from build123d import *

# Parameters (mm, degrees)
BOSS_EXTRU_1_DEPTH      = 20
ESQUISSE2_W             = 4.75
ESQUISSE2_H             = 4.5
ENL_V_MAT_EXTRU_1_DEPTH = 21
ESQUISSE3_W             = 4.75
ESQUISSE3_H             = 4.5
ENL_V_MAT_EXTRU_2_DEPTH = 21


with BuildPart() as part:
    # Esquisse1 → Boss.-Extru.1 (new body)
    with BuildSketch(Plane(origin=(0, 0, -10), x_dir=(-1, 0, 0), z_dir=(0, 0, -1))):
        Polygon((9.75, -1.5), (9.75, 5), (-9.75, 5), (-9.75, -1.5), (-6.25, -5), (6.25, -5), align=None)
    extrude(amount=-BOSS_EXTRU_1_DEPTH)

    # Esquisse2 → Enlèv. mat.-Extru.1 (cut, through all)
    with BuildSketch(Plane(origin=(0, 0, -10), x_dir=(-1, 0, 0), z_dir=(0, 0, -1))):
        with Locations((-7.375, 2.75)):
            Rectangle(ESQUISSE2_W, ESQUISSE2_H)
    extrude(amount=-ENL_V_MAT_EXTRU_1_DEPTH, mode=Mode.SUBTRACT)

    # Esquisse3 → Enlèv. mat.-Extru.2 (cut, through all)
    with BuildSketch(Plane(origin=(0, 0, -10), x_dir=(-1, 0, 0), z_dir=(0, 0, -1))):
        with Locations((7.375, 2.75)):
            Rectangle(ESQUISSE3_W, ESQUISSE3_H)
    extrude(amount=-ENL_V_MAT_EXTRU_2_DEPTH, mode=Mode.SUBTRACT)

    # Esquisse4 → Enlèvement de matière-Révolution1 (revolve, cut)
    with BuildSketch(Plane.XY):
        Polygon((3, 5), (0, 5), (0, -5), (3, -5), (2.4585, -4.4585), (2.4585, 4.4585), align=None)
    revolve(axis=Axis((0, 5, 0), (0, -1, 0)), mode=Mode.SUBTRACT)


solid = part.part
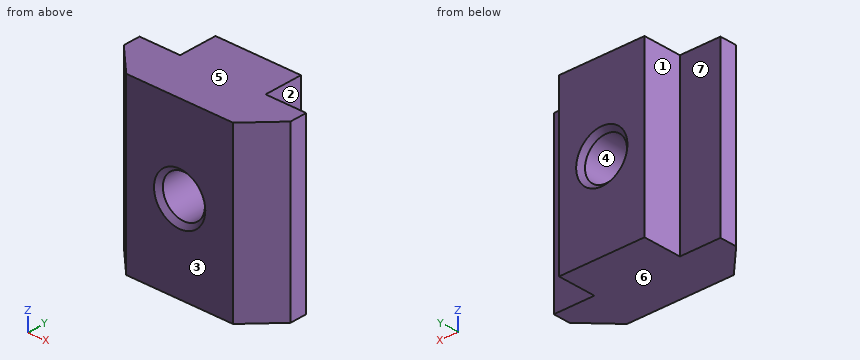
Verification items for the finished model (mm, model axes). Face numbers are marked on the shaded views. A direction names the side the tool comes from. Give positions to 0.01 mm unless a question says otherwise; leave off trailing zeros. Order: outer loops, then holes, each group sorted by start corner. A loop starts at its lowest first (then second) coordinate and runs counter-clockwise, first axis right, second up. Notation, with made-up numbers: M 31.5,71.25 L 83.5,71.25 A13 ccw 83.5,76.25 Z; hole C 49.5,59.25 d4. An arc over 180 degrees is marked long. Answer as a JSON object with one key per item and string values. Group by question number.
1) Depth check by flat-ended pin: pin 1 Ø2 at (x, z) = (-6.5, 4) entering from +Y. Enter the tip coordinate at first touch or a pass-through.
2) Cross-section at A-A (x = 0). Enter the section's corners in (y, z).
3) Cross-section at C-C (y = -0.75). Enter the section's corners in (x, z).
4) Access from +Z, -Z, +X, -X, +Y, -Y to the whole of each face (thin tool, end or side, straight path). Record for the marked faces 1, 2 and 3.
5) Mould release check, pull along Z, two halves, no side actions. Record for the marked faces 4, 5, 6 and 7: released by +Z, released by -Z, zero draft, split by the parting line, or undercut.
6) Scan lines: line 1 along Z through (x, y) = (0, 1.5); line 2 along X through (y, z) = (0.75, -4.75); line 3 along X through (y, z) = (-2.5, 1.5). Record each from-to range of solid material in increasing order. Write a range as [from, to].
7) Cross-section at D-D (z = -8.5). Enter the section's corners in (x, y).
8) Cross-section at B-B (z = 0). Enter the section's corners in (x, y).
Result sheet:
{
 "1": {"pin 1": "stops at y = 0.5"},
 "2": {"outline": "M -5,-10 L 5,-10 L 5,-3 L 4.46,-2.46 L -4.46,-2.46 L -5,-3 Z; M -5,3 L -4.46,2.46 L 4.46,2.46 L 5,3 L 5,10 L -5,10 Z"},
 "3": {"outline": "M -9.75,-10 L 9.75,-10 L 9.75,10 L -9.75,10 Z; hole C 0,0 d4.92"},
 "4": {"face 1": "+Z, -Z, -X, +Y", "face 2": "+Z, -Z, +X, +Y", "face 3": "+Z, -Z, +X, -X, -Y"},
 "5": {"face 4": "undercut", "face 5": "released by +Z", "face 6": "released by -Z", "face 7": "zero draft"},
 "6": {"line 1": "z = [-10, -2.46], [2.46, 10]", "line 2": "x = [-5, 5]", "line 3": "x = [-8.75, -1.95], [1.95, 8.75]"},
 "7": {"outline": "M -9.75,-1.5 L -6.25,-5 L 6.25,-5 L 9.75,-1.5 L 9.75,0.5 L 5,0.5 L 5,5 L -5,5 L -5,0.5 L -9.75,0.5 Z"},
 "8": {"outline": "M -9.75,-1.5 L -6.25,-5 L -3,-5 L -2.46,-4.46 L -2.46,4.46 L -3,5 L -5,5 L -5,0.5 L -9.75,0.5 Z; M 2.46,-4.46 L 3,-5 L 6.25,-5 L 9.75,-1.5 L 9.75,0.5 L 5,0.5 L 5,5 L 3,5 L 2.46,4.46 Z"}
}
